from build123d import *

# Parameters (mm, degrees)
F0_W     = 48.4505593777
F0_H     = 45.2879294753
F1_DEPTH = 350
F2_DEPTH = 18
F3_DEPTH = 600
F4_DEPTH = 400
F5_T     = -18
F6_R     = 2
F7_R     = 2


with BuildPart() as f1:
    # F0 (on Front) → F1 (new body)
    with BuildSketch(Plane.XZ):
        with Locations((24.2252796888, 22.6439647377)):
            Rectangle(F0_W, F0_H)
    extrude(amount=F1_DEPTH)

    # F2 (intersect): a face of the model
    f2_faces = [f1.faces().sort_by_distance(p)[0] for p in [
        (0, -175, 22.6439647377),
    ]]
    extrude(f2_faces, amount=-F2_DEPTH, mode=Mode.INTERSECT)

    # F3 (add): a face of the model
    f3_faces = [f1.faces().sort_by_distance(p)[0] for p in [
        (9, -175, 0),
    ]]
    extrude(f3_faces, amount=-F3_DEPTH)

    # F4 (add): a face of the model
    f4_faces = [f1.faces().sort_by_distance(p)[0] for p in [
        (0, -175, 300),
    ]]
    extrude(f4_faces, amount=-F4_DEPTH)

    # F5
    f5_openings = [f1.faces().sort_by_distance(p)[0] for p in [
        (200, -350, 300),
        (200, -175, 0),
    ]]
    offset(amount=F5_T, openings=f5_openings)

    # F6
    f6_edges = [f1.edges().sort_by_distance(p)[0] for p in [
        (400, -350, 300),
        (200, -350, 600),
        (0, -350, 300),
    ]]
    fillet(f6_edges, radius=F6_R)

    # F7
    f7_edges = [f1.edges().sort_by_distance(p)[0] for p in [
        (18, -350, 291),
        (382, -350, 291),
        (200, -350, 582),
    ]]
    fillet(f7_edges, radius=F7_R)


solid = f1.part
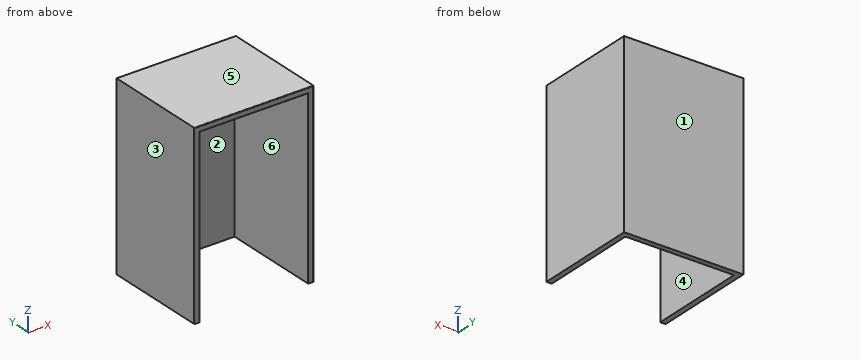
Geometry check sheet. Reference: the model listing, model coordinates, mm. Face numbers are marked on the shaded views. A direction names the side the tool comes from. Give positions to 0.01 mm unless a question says otherwise; leave off trailing zeros. Order: outer loops, then holes, each group sorted by start corner. A loop starts at its lowest first (then second) coordinate and runs counter-clockwise, first axis right, second up. Notation, with made-up numbers: (34, 45) - (42, 45) arc R19 ccw to (42, 66) - close; hole circle Ø7 at (70.25, 21.5). An arc over 180 degrees is marked (long way). Answer as a JSON object with one key per item and string values.
(1) Cross-section at B-B (z = 118). Record the cut outline in (x, y), then the cut area to 3 significant figures.
Report:
{"outline": "(0, -348) arc R2 ccw to (2, -350) - (16, -350) arc R2 ccw to (18, -348) - (18, -18) - (382, -18) - (382, -348) arc R2 ccw to (384, -350) - (398, -350) arc R2 ccw to (400, -348) - (400, 0) - (0, 0) - close", "area": "19,100 mm^2"}
(2) Tool access check on the marked faces 1 and 2. Record the directions out of +Z, -Z, +X, -X, +Y, -Y that give a thin tool (end or side, any length) a straight path to the whole face; none if there is none.
Report:
{"face 1": "+Z, -Z, +X, -X, +Y", "face 2": "-Z, -Y"}
(3) Depth check by flat-ended pin: pin 1 Ø12 at (x, y) = (105, -211.5) entering from -Z; pin 2 Ø6 at (x, z) = (272.5, 310.5) entering from -Y. Enter the tip coordinate at first touch or a pass-through.
Report:
{"pin 1": "z = 582", "pin 2": "y = -18"}
(4) Draft check along X on the marked faces 3, 4, 5 and 6. Enter one of: released by +X, released by -X, zero draft, split by the parting line, or undercut.
Report:
{"face 3": "released by -X", "face 4": "undercut", "face 5": "zero draft", "face 6": "undercut"}
(5) Material ranges on line 1 (X direction, y = -319, z = 535); line 2 (Z direction, x = 350, y = -299); line 3 (Y direction, x = 179, z = 122), recorded low to high.
Report:
{"line 1": "0 to 18, 382 to 400", "line 2": "582 to 600", "line 3": "-18 to 0"}
(6) Cross-section at C-C (y = -51). Record the cut outline in (x, z), then the cut area to 3 significant figures.
Report:
{"outline": "(0, 0) - (18, 0) - (18, 582) - (382, 582) - (382, 0) - (400, 0) - (400, 600) - (0, 600) - close", "area": "28,200 mm^2"}
(7) Cross-section at A-A (x = 195). Record the cut outline in (y, z).
Report:
{"outline": "(-350, 584) arc R2 ccw to (-348, 582) - (-18, 582) - (-18, 0) - (0, 0) - (0, 600) - (-348, 600) arc R2 ccw to (-350, 598) - close"}
